Can you work these out from the drawing? Everything is in mm from the part's minimum corner. Round coordinates to 2 decimals unless told otherwise and drop trailing zeros. Loops run counter-clockwise (first coordinate to the right, second up) from the corner with the lowest first, then second, coordinate; pieces in that order, holes last. Notation, with made-up numbers: (-16, 44) -> (-4, 44) arc R27 cw to (-4, 69) -> close; hole circle Ø9 at (-23.75, 47). An arc over 180 degrees is marked (long way). One line per item, written item: value.
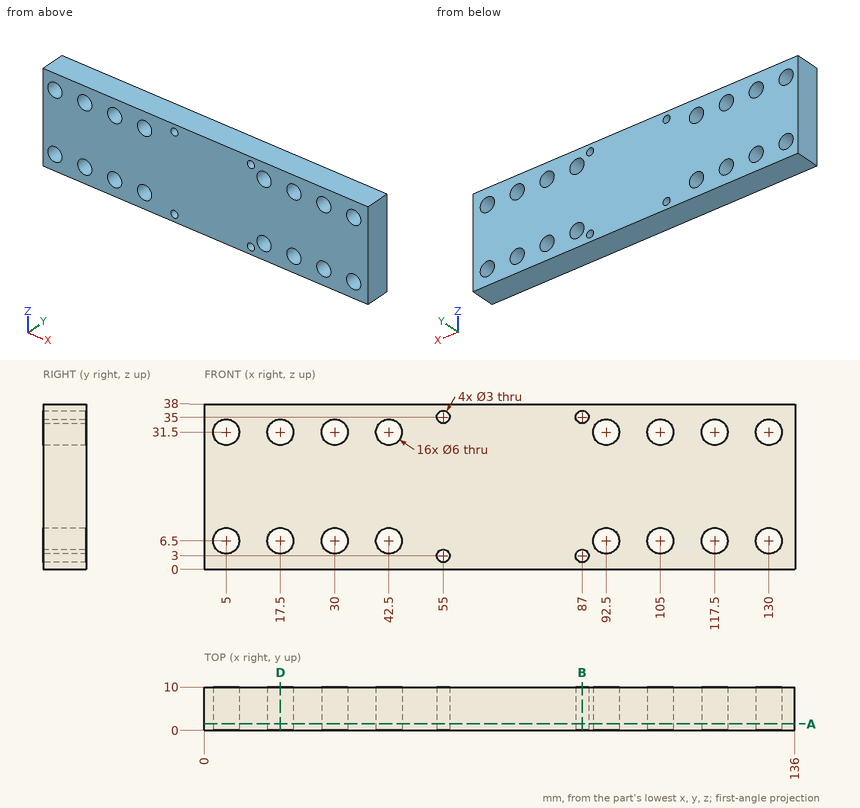
(1) If I drill on L1, parallel to Z at x = 16, y = 2.25; L2, parallel to X at y = 4.5, z = 2, over which ranges is the centre line in solid material (lowest first)?
Recorded:
L1: 0 to 3.9, 9.1 to 28.9, 34.1 to 38
L2: 0 to 53.88, 56.12 to 85.88, 88.12 to 136
(2) I'm going to push a flat-ended pin straight in: pin 1 Ø3.5 at (x, z) = (17.5, 31.5) entering from +Y. Where does the tip first touch, or does it pass through?
Recorded:
pin 1: through
(3) If we section it at B-B, the plane x = 87: Please give me the cut outline in (y, z).
Recorded:
outline: (0, 0) -> (10, 0) -> (10, 1.5) -> (0, 1.5) -> close; (0, 4.5) -> (10, 4.5) -> (10, 33.5) -> (0, 33.5) -> close; (0, 36.5) -> (10, 36.5) -> (10, 38) -> (0, 38) -> close
(4) If we section it at A-A, the plane y = 1.5: Give the number of separate pieces and of enclosed holes in the cut face, then the cut area to 3 significant figures.
Recorded:
separate pieces: 1
enclosed holes: 20
area: 4,690 mm²
(5) If we section it at D-D, the plane x = 17.5: Please give me the cut outline in (y, z).
Recorded:
outline: (0, 0) -> (10, 0) -> (10, 3.5) -> (0, 3.5) -> close; (0, 9.5) -> (10, 9.5) -> (10, 28.5) -> (0, 28.5) -> close; (0, 34.5) -> (10, 34.5) -> (10, 38) -> (0, 38) -> close
